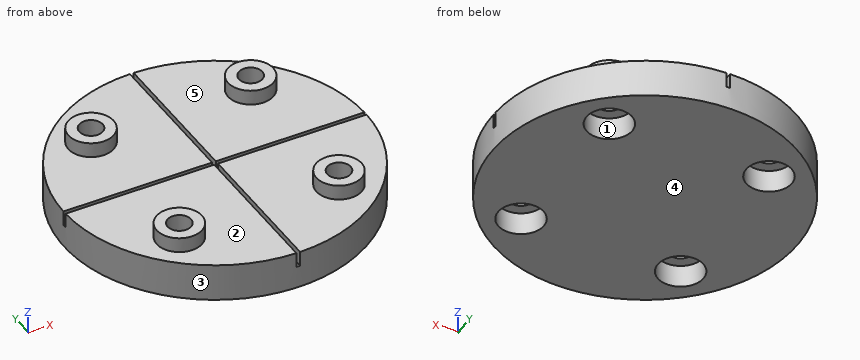
from build123d import *

# Parameters (mm, degrees)
F0_R     = 20
F1_DEPTH = 5
F2_W     = 0.5
F2_H     = 21.0267571211
F2_H_2   = 0.5
F2_W_2   = 21.8651188016
F2_W_3   = 23.3558980227
F2_H_3   = 21.8529557288
F3_DEPTH = 2
F5_R     = 3
F6_DEPTH = 7
F7_DEPTH = 3
F4_R     = 1.55
F8_DEPTH = 5.001
F9_DEPTH = 2.001


with BuildPart() as f1:
    # F0 (on Top) → F1 (new body)
    with BuildSketch(Plane.XY):
        Circle(F0_R)
    extrude(amount=F1_DEPTH)

    # F2 (on face) → F3 (cut)
    with BuildSketch(Plane.XY.offset(5)):
        with Locations((0, 10.7633785605)):
            Rectangle(F2_W, F2_H)
        Rectangle(F2_W, F2_H_2)
        with Locations((-11.1825594008, 0)):
            Rectangle(F2_W_2, F2_H_2)
        with Locations((11.9279490113, 0)):
            Rectangle(F2_W_3, F2_H_2)
        with Locations((0, -11.1764778644)):
            Rectangle(F2_W, F2_H_3)
    extrude(amount=-F3_DEPTH, mode=Mode.SUBTRACT)

    # F5 (on face) → F6 (join)
    with BuildSketch(Plane(origin=(0, 0, 0), x_dir=(1, 0, 0), z_dir=(0, 0, -1))):
        with Locations((-10.6066017178, 10.6066017178)):
            Circle(F5_R)
        with Locations((10.6066017178, 10.6066017178)):
            Circle(F5_R)
        with Locations((10.6066017178, -10.6066017178)):
            Circle(F5_R)
        with Locations((-10.6066017178, -10.6066017178)):
            Circle(F5_R)
    extrude(amount=-F6_DEPTH)

    # F5 (on face) → F7 (cut)
    with BuildSketch(Plane(origin=(0, 0, 0), x_dir=(1, 0, 0), z_dir=(0, 0, -1))):
        with Locations((-10.6066017178, 10.6066017178)):
            Circle(F5_R)
        with Locations((10.6066017178, 10.6066017178)):
            Circle(F5_R)
        with Locations((10.6066017178, -10.6066017178)):
            Circle(F5_R)
        with Locations((-10.6066017178, -10.6066017178)):
            Circle(F5_R)
    extrude(amount=-F7_DEPTH, mode=Mode.SUBTRACT)

    # F4 (on face) → F8 (cut, through all)
    with BuildSketch(Plane.XY.offset(5)):
        with Locations((10.6066017178, -10.6066017178)):
            Circle(F4_R)
        with Locations((10.6066017178, 10.6066017178)):
            Circle(F4_R)
        with Locations((-10.6066017178, 10.6066017178)):
            Circle(F4_R)
        with Locations((-10.6066017178, -10.6066017178)):
            Circle(F4_R)
    extrude(amount=-F8_DEPTH, mode=Mode.SUBTRACT)

    # F4 (on face) → F9 (cut, through all)
    with BuildSketch(Plane.XY.offset(5)):
        with Locations((10.6066017178, -10.6066017178)):
            Circle(F4_R)
        with Locations((10.6066017178, 10.6066017178)):
            Circle(F4_R)
        with Locations((-10.6066017178, 10.6066017178)):
            Circle(F4_R)
        with Locations((-10.6066017178, -10.6066017178)):
            Circle(F4_R)
    extrude(amount=F9_DEPTH, mode=Mode.SUBTRACT)


solid = f1.part
For this review, take the finished solid that the model builds, in its own axes (mm). Face numbers are marked on the shaded views. A direction names the side the tool comes from. Coordinates: 2 decimals unless noted, no trailing zeros. Loops run counter-clockwise (first coordinate to the right, second up) from the corner with the lowest first, then second, coordinate; pieces in that order, holes last. Notation, with made-up numbers: (26.5, 43.25) -> (43.5, 43.25) arc R18 ccw to (43.5, 66.25) -> close; hole circle Ø10 at (27, 22). An arc over 180 degrees is marked (long way). Write each question's results on one line, items separated by ' | '.
Q1. To check wall thickness, follow line 1 along X through (y, z) = (9.5, 3.75); line 2 along X through (y, z) = (-10, 3.25); line 3 along Y through (x, z) = (10, 5.5). State the ranges of each line that lie inside material, in increasing order. Write a range as [from, to].
Taken from the geometry:
line 1: [-17.6, -11.69], [-9.52, -0.25], [0.25, 9.52], [11.69, 17.6] | line 2: [-17.32, -12.03], [-9.18, -0.25], [0.25, 9.18], [12.03, 17.32] | line 3: [-13.54, -12.03], [-9.18, -7.67], [7.67, 9.18], [12.03, 13.54]
Q2. For pin 1 Ø2 at (y, z) = (13, 4) entering from -X; pin 2 Ø1.5 at (y, z) = (3, 2) entering from -X; pin 3 Ø2 at (x, z) = (8, 4.5) entering from -Y (3 decimals), all flat-tipped, find the tip position at first contact; note any pin that passes through.
Taken from the geometry:
pin 1: x = -16 | pin 2: x = -19.87 | pin 3: y = -18.735
Q3. Add section A-A, the plane x = -10.5. Count the separate pieces of the cut face and the enclosed holes in it, then the cut area to 3 significant figures.
Taken from the geometry:
separate pieces: 3 | enclosed holes: 0 | area: 132 mm²
Q4. Mouldability with a two-part tool opening along Y and no side actions: class the marked faces 3, 4 and 5 as +Y half, -Y half, draft (parallel to the pull), parting line (faces both ways), or undercut.
Taken from the geometry:
face 3: parting line | face 4: draft | face 5: undercut
Q5. Add section D-D, the plane z = 2.5. State the section outline as (x, y) points.
Taken from the geometry:
outline: circle Ø40 at (0, 0); hole circle Ø6 at (-10.61, -10.61); hole circle Ø6 at (-10.61, 10.61); hole circle Ø6 at (10.61, -10.61); hole circle Ø6 at (10.61, 10.61)
Q6. Machinability: for the marked faces 1 and 2, which of the approach directions +Z, -Z, +X, -X, +Y, -Y give a long, thin tool a straight path to every point of the face, cutting with its end or side? Answer none if there is none.
Taken from the geometry:
face 1: -Z | face 2: +Z
Q7. Add section B-B, the plane x = -6.5. State the section outline as (y, z) points.
Taken from the geometry:
outline: (-18.91, 0) -> (18.91, 0) -> (18.91, 5) -> (0.25, 5) -> (0.25, 3) -> (-0.25, 3) -> (-0.25, 5) -> (-18.91, 5) -> close
Q8. Add section C-C, the plane y = 5. State the section outline as (x, z) points, then the cut area to 3 significant figures.
Taken from the geometry:
outline: (-19.36, 0) -> (19.36, 0) -> (19.36, 5) -> (0.25, 5) -> (0.25, 3) -> (-0.25, 3) -> (-0.25, 5) -> (-19.36, 5) -> close | area: 193 mm²
